The listing builds one solid part. Answer for the finished solid, in the listing's coordinates (mm). A direction names the side the tool comes from. Round coordinates to 2 decimals unless told otherwise and drop trailing zeros. Loops run counter-clockwise (first coordinate to the right, second up) from the corner with the lowest first, then second, coordinate; pieces in that order, holes last. Notation, with made-up numbers: (10.25, 28) - (63.25, 28) arc R28 ccw to (63.25, 55) - close; hole circle Ø4 at (51.25, 11). An arc over 180 degrees is marked (long way). Write item = value, one per line. Start each with the question number.
1) A tool of negligible diameter and unlimited length cuts with its end or side. For faces 4 (the flat face through (-9.5, 40, 19)), 5 (the flat face through (9.5, 40, 19)), 6 (the flat face through (14.5, 24, 7)), from which of +Z, -Z, +X, -X, +Y, -Y can it reach the whole face along a straight path? Write none if from no direction.
2) Given pin 1 Ø12 at (y, z) = (18, 12) entering from +X; pin 2 Ø5 at (x, z) = (19, 10) entering from +Y; pin 3 Ø12 at (x, z) = (-1.5, 15.5) entering from -Y; pin 4 Ø2 at (x, z) = (-20, 7.52) entering from -Y, each flat-ended and moving along its own axis, determine where each tip first touches the part or whether it passes through.
3) Section C-C, the plane z = 21 is taken. Determine the outline of the cut face in (x, y), and give its area (3 significant figures).
4) Section B-B, the plane x = -21 is taken. Determine the outline of the cut face in (y, z).
5) For a pull along X with two mould halves and no side action, classify faces 1 (the cylindrical face through (8, 36.57, 7.1)), 2 (the flat face through (0, 43, 12)), 3 (the flat face through (-14.5, 24, 7)) as released by +X, released by -X, zero draft, split by the parting line, or undercut.
6) Section A-A, the plane y = 23.5 is taken. Determine the outline of the cut face in (x, z).
7) Straight lines are drawn through the part: line 1 along X through (y, z) = (21.5, 1.75); line 2 along Z through (x, y) = (-20, 4); line 3 along Y through (x, z) = (-3, 2.75). For each, find the intervals that lie inside material, in ascending order.
from build123d import *

# Parameters (mm, degrees)
BOSS_EXTRUDE1_DEPTH     = 14
FILLET1_R               = 5
FILLET2_R               = 5
CUT_EXTRUDE3_DEPTH      = 10
CUT_EXTRUDE3_DEPTH_BACK = 10
SKETCH2_R               = 1.636049027
SKETCH4_W               = 19
SKETCH4_H               = 5
BOSS_EXTRUDE2_DEPTH     = 10
SKETCH5_R               = 2.5
CUT_EXTRUDE4_DEPTH      = 10


with BuildPart() as part:
    # Sketch1 → Boss-Extrude1 (new body)
    with BuildSketch(Plane.XY):
        Polygon((-24.5, 0), (-24.5, 5), (-14.5, 5), (-14.5, 43), (14.5, 43), (14.5, 5), (24.5, 5), (24.5, 0), (9.5, 0), (9.5, 38), (-9.5, 38), (-9.5, 0), align=None)
    extrude(amount=BOSS_EXTRUDE1_DEPTH)

    # Fillet1
    fillet1_edges = [part.edges().sort_by_distance(p)[0] for p in [
        (-14.5, 43, 7),
        (14.5, 43, 7),
        (24.5, 5, 7),
        (-24.5, 5, 7),
        (14.5, 5, 7),
        (-14.5, 5, 7),
    ]]
    fillet(fillet1_edges, radius=FILLET1_R - 0.0001)  # a hair under: the kernel refuses the full size

    # Fillet2
    fillet2_edges = [part.edges().sort_by_distance(p)[0] for p in [
        (9.5, 38, 7),
        (-9.5, 38, 7),
    ]]
    fillet(fillet2_edges, radius=FILLET2_R)

    # Sketch2 → Cut-Extrude3 (cut, two sides: drawn at the far end of the back side and taken through both)
    with BuildSketch(Plane(origin=(0, 0, 0), x_dir=(1, 0, 0), z_dir=(0, 1, 0)).offset(-CUT_EXTRUDE3_DEPTH_BACK)):
        with Locations(Location((-20, -7.523321805, 0), (0, 0, 72.20487372))):
            Circle(SKETCH2_R)
        with Locations(Location((20, -7.523321805, 0), (0, 0, 107.795126278))):
            Circle(SKETCH2_R)
    extrude(amount=CUT_EXTRUDE3_DEPTH + CUT_EXTRUDE3_DEPTH_BACK, mode=Mode.SUBTRACT)

    # Sketch4 → Boss-Extrude2 (add)
    with BuildSketch(Plane.XY.offset(14)):
        with Locations((0, 40.5)):
            Rectangle(SKETCH4_W, SKETCH4_H)
    extrude(amount=BOSS_EXTRUDE2_DEPTH)

    # Sketch5 → Cut-Extrude4 (cut)
    with BuildSketch(Plane(origin=(0, 43, 0), x_dir=(1, 0, 0), z_dir=(0, 1, 0))):
        with Locations(Location((4.70575, -19.60149527, 0), (0, 0, 270))):
            Circle(SKETCH5_R)
        with Locations(Location((-5.477408827, -19.618067384, 0), (0, 0, 270))):
            Circle(SKETCH5_R)
    extrude(amount=-CUT_EXTRUDE4_DEPTH, mode=Mode.SUBTRACT)


solid = part.part
Geometry check:
q1.face_4 = +Z, -X, +Y, -Y
q1.face_5 = +Z, +X, +Y, -Y
q1.face_6 = +Z, -Z, +X, +Y
q2.pin_1 = 14.5
q2.pin_2 = 6
q2.pin_3 = 37.14
q2.pin_4 = through
q3.outline = (-9.5, 38) - (-7.56, 38) - (-7.56, 43) - (-9.5, 43) - close; (-3.39, 38) - (2.63, 38) - (2.63, 43) - (-3.39, 43) - close; (6.78, 38) - (9.5, 38) - (9.5, 43) - (6.78, 43) - close
q3.area = 53.4 mm2
q4.outline = (0, 0) - (4.77, 0) - (4.77, 6.23) - (0, 6.23) - close; (0, 8.82) - (4.77, 8.82) - (4.77, 14) - (0, 14) - close
q5.face_1 = undercut
q5.face_2 = zero draft
q5.face_3 = released by -X
q6.outline = (-14.5, 0) - (-9.5, 0) - (-9.5, 14) - (-14.5, 14) - close; (9.5, 0) - (14.5, 0) - (14.5, 14) - (9.5, 14) - close
q7.line_1 = -14.5 to -9.5, 9.5 to 14.5
q7.line_2 = 0 to 5.89, 9.16 to 14
q7.line_3 = 38 to 43
